Design review of the part built by this model. Coordinates are the model's own, in mm. A direction names the side the tool comes from. Coordinates: 2 decimals unless noted, no trailing zeros. Loops run counter-clockwise (first coordinate to the right, second up) from the corner with the lowest first, then second, coordinate; pieces in that order, holes last. Notation, with made-up numbers: (19, 33.5) -> (49, 33.5) arc R16 ccw to (49, 39.5) -> close; hole circle Ø9 at (14, 4.5). An arc over 180 degrees is marked (long way). Answer in a Markdown table with one row per item.
```python
from build123d import *

# Parameters (mm, degrees)
BOSS_EXTRUDE1_DEPTH = 40
SKETCH4_R           = 6
CUT_EXTRUDE1_DEPTH  = 71.710678119
CUT_EXTRUDE2_DEPTH  = 1


with BuildPart() as part:
    # Sketch1 → Boss-Extrude1 (new body)
    with BuildSketch(Plane.XY):
        Polygon((0, 0), (0, 30), (2, 30), (2, 2), (50, 2), (50, 0), align=None)
    extrude(amount=BOSS_EXTRUDE1_DEPTH)

    # Sketch4 → Cut-Extrude1 (cut, through all)
    with BuildSketch(Plane(origin=(0, 0, 0), x_dir=(-1, 0, 0), z_dir=(0, -1, 0))):
        with BuildLine():
            Line((-50, -26), (-35, -26))
            ThreePointArc((-35, -26), (-41, -20), (-35, -14))
            Line((-35, -14), (-50, -14))
            Line((-50, -14), (-50, -26))
        make_face()
        with Locations((-35, -20)):
            Circle(SKETCH4_R)
    extrude(amount=-CUT_EXTRUDE1_DEPTH, mode=Mode.SUBTRACT)

    # Sketch5 → Cut-Extrude2 (cut)
    with BuildSketch(Plane(origin=(0, 0, 0), x_dir=(-1, 0, 0), z_dir=(0, -1, 0))):
        with BuildLine():
            Line((-50, -30), (-35, -30))
            ThreePointArc((-35, -30), (-39.472135955, -28.94427191), (-43, -26))
            Line((-43, -26), (-50, -26))
            Line((-50, -26), (-50, -30))
        make_face()
        with BuildLine():
            Line((-50, -14), (-43, -14))
            ThreePointArc((-43, -14), (-39.876214832, -11.269448533), (-35.913040721, -10.041769402))
            Line((-35.913040721, -10.041769402), (-50, -10))
            Line((-50, -10), (-50, -14))
        make_face()
        with BuildLine():
            ThreePointArc((-43, -26), (-39.472135955, -28.94427191), (-35, -30))
            ThreePointArc((-35, -30), (-27.928932188, -27.071067812), (-25, -20))
            ThreePointArc((-25, -20), (-27.593219771, -13.281398461), (-34.027921329, -10.047358991))
            Line((-34.027921329, -10.047358991), (-35.913040721, -10.041769402))
            ThreePointArc((-35.913040721, -10.041769402), (-39.876214832, -11.269448533), (-43, -14))
            Line((-43, -14), (-35, -14))
            ThreePointArc((-35, -14), (-29, -20), (-35, -26))
            Line((-35, -26), (-43, -26))
        make_face()
    extrude(amount=-CUT_EXTRUDE2_DEPTH, mode=Mode.SUBTRACT)


solid = part.part
```
(1) Take a section at D-D on z = 17.5. Give the boundary of the cut face in (x, y), and give its area (3 significant figures).
Evaluation:
| item | result |
|---|---|
| outline | (0, 0) -> (25.32, 0) -> (25.32, 1) -> (29.55, 1) -> (29.55, 2) -> (2, 2) -> (2, 30) -> (0, 30) -> close |
| area | 111 mm² |
(2) Take a section at B-B on y = 27.25. Give the boundary of the cut face in (x, z), and give its area (3 significant figures).
Evaluation:
| item | result |
|---|---|
| outline | (0, 0) -> (2, 0) -> (2, 40) -> (0, 40) -> close |
| area | 80.0 mm² |
(3) Draft analysis for pull direction Z (two halves, no side actions). For faces 4 (the cylindrical face through (29, 1.5, 20.1)), 5 (the flat face through (17.7, 1.7, 40)), 6 (the flat face through (0, 15, 20)), state which applies: pulls with the +Z half, pulls with the -Z half, needs draft (parallel to the pull), parting line crosses it, or undercut.
Evaluation:
| item | result |
|---|---|
| face 4 | undercut |
| face 5 | pulls with the +Z half |
| face 6 | needs draft |
(4) Tool access review of faces 1 (the flat face through (26, 2, 20)), 2 (the flat face through (20, 0, 20)), 3 (the flat face through (38, 1, 13)): name each direction out of +Z, -Z, +X, -X, +Y, -Y from which nothing blocks a thin tool from reaching the whole face with its end or side.
Evaluation:
| item | result |
|---|---|
| face 1 | +Z, -Z, +X, +Y |
| face 2 | +Z, -Z, +X, -X, -Y |
| face 3 | +X, -Y |
(5) For pin 1 (4 mm diameter, centred on x = 13.5, z = 8, fed in from +Y); pin 2 (12 mm diameter, centred on y = 16, z = 19, fed in from +X); pin 3 (6 mm diameter, centred on x = 33, z = 16, fed in from -Y), all flat-tipped, find the tip position at first contact; note any pin that passes through.
Evaluation:
| item | result |
|---|---|
| pin 1 | stops at y = 2 |
| pin 2 | stops at x = 2 |
| pin 3 | stops at y = 1 |
(6) Take a section at A-A on z = 12. Give the boundary of the cut face in (x, y), and give its area (3 significant figures).
Evaluation:
| item | result |
|---|---|
| outline | (0, 0) -> (29, 0) -> (29, 1) -> (50, 1) -> (50, 2) -> (2, 2) -> (2, 30) -> (0, 30) -> close |
| area | 135 mm² |
(7) To check wall thickness, follow probe 1 along X at (y, z) = (10, 20.5); probe 2 along Y at (x, z) = (27, 22.5). State the ranges of each line that lie inside material, in increasing order.
Evaluation:
| item | result |
|---|---|
| probe 1 | x = 0 to 2 |
| probe 2 | y = 1 to 2 |
